CAD build for the part. Positions are in the model's coordinates, mm. A direction names the side the tool comes from. Round coordinates to 2 decimals unless told otherwise and drop trailing zeros. Loops run counter-clockwise (first coordinate to the right, second up) from the corner with the lowest first, then second, coordinate; pieces in that order, holes last.
```python
from build123d import *

# Parameters (mm, degrees)
BOSS_EXTRUDE1_DEPTH = 50
SKETCH2_W           = 3
SKETCH2_H           = 45
CUT_EXTRUDE1_DEPTH  = 50
SKETCH3_W           = 2
SKETCH3_H           = 45
CUT_EXTRUDE2_DEPTH  = 83.643814046
SKETCH4_W           = 3
SKETCH4_H           = 2
BOSS_EXTRUDE2_DEPTH = 39
SKETCH5_W           = 8
SKETCH5_H           = 2
BOSS_EXTRUDE3_DEPTH = 39
CUT_EXTRUDE3_REACH  = 83.222
SKETCH6_R           = 2.5


with BuildPart() as part:
    # Sketch1 → Boss-Extrude1 (new body)
    with BuildSketch(Plane.XY):
        Polygon((-8, 8), (53, 8), (53, -31), (-8, -31), (-8, -23.5), (-8, 0.5), align=None)
        Polygon((0, 0), (45, 0), (45, -23), (0, -23), (0, -15.5), (-3, -15.5), (-3, -7.5), (0, -7.5), align=None, mode=Mode.SUBTRACT)
    extrude(amount=BOSS_EXTRUDE1_DEPTH)

    # Sketch2 → Cut-Extrude1 (cut)
    with BuildSketch(Plane(origin=(0, 8, 0), x_dir=(1, 0, 0), z_dir=(0, 1, 0))):
        with Locations((-6.5, -24.5)):
            Rectangle(SKETCH2_W, SKETCH2_H)
        with Locations((51.5, -24.5)):
            Rectangle(SKETCH2_W, SKETCH2_H)
    extrude(amount=-CUT_EXTRUDE1_DEPTH, mode=Mode.SUBTRACT)

    # Sketch3 → Cut-Extrude2 (cut, through all)
    with BuildSketch(Plane(origin=(0, 8, 0), x_dir=(1, 0, 0), z_dir=(0, 1, 0))):
        with Locations((49, -24.5)):
            Rectangle(SKETCH3_W, SKETCH3_H)
    extrude(amount=-CUT_EXTRUDE2_DEPTH, mode=Mode.SUBTRACT)

    # Sketch4 → Boss-Extrude2 (add)
    with BuildSketch(Plane(origin=(0, 8, 0), x_dir=(1, 0, 0), z_dir=(0, 1, 0))):
        with Locations((54.5, -1)):
            Rectangle(SKETCH4_W, SKETCH4_H)
    extrude(amount=-BOSS_EXTRUDE2_DEPTH)

    # Sketch5 → Boss-Extrude3 (add)
    with BuildSketch(Plane(origin=(0, 8, 0), x_dir=(1, 0, 0), z_dir=(0, 1, 0))):
        with Locations((-9, -1)):
            Rectangle(SKETCH5_W, SKETCH5_H)
    extrude(amount=-BOSS_EXTRUDE3_DEPTH)

    # Sketch6 → Cut-Extrude3 (cut, up to next)
    with BuildSketch(Plane(origin=(0, 0, 0), x_dir=(-1, 0, 0), z_dir=(0, 0, -1)), mode=Mode.PRIVATE) as cut_extrude3_sk1:
        with Locations((-52, -1.5)):
            Circle(SKETCH6_R)
    cut_extrude3_tool1 = extrude(cut_extrude3_sk1.sketch, amount=-CUT_EXTRUDE3_REACH, mode=Mode.PRIVATE) & part.part
    # Sketch6 → Cut-Extrude3 (cut, up to next)
    with BuildSketch(Plane(origin=(0, 0, 0), x_dir=(-1, 0, 0), z_dir=(0, 0, -1)), mode=Mode.PRIVATE) as cut_extrude3_sk2:
        with Locations((-52, -21.5)):
            Circle(SKETCH6_R)
    cut_extrude3_tool2 = extrude(cut_extrude3_sk2.sketch, amount=-CUT_EXTRUDE3_REACH, mode=Mode.PRIVATE) & part.part
    # Sketch6 → Cut-Extrude3 (cut, up to next)
    with BuildSketch(Plane(origin=(0, 0, 0), x_dir=(-1, 0, 0), z_dir=(0, 0, -1)), mode=Mode.PRIVATE) as cut_extrude3_sk3:
        with Locations((9, -21.5)):
            Circle(SKETCH6_R)
    cut_extrude3_tool3 = extrude(cut_extrude3_sk3.sketch, amount=-CUT_EXTRUDE3_REACH, mode=Mode.PRIVATE) & part.part
    # Sketch6 → Cut-Extrude3 (cut, up to next)
    with BuildSketch(Plane(origin=(0, 0, 0), x_dir=(-1, 0, 0), z_dir=(0, 0, -1)), mode=Mode.PRIVATE) as cut_extrude3_sk4:
        with Locations((9, -1.5)):
            Circle(SKETCH6_R)
    cut_extrude3_tool4 = extrude(cut_extrude3_sk4.sketch, amount=-CUT_EXTRUDE3_REACH, mode=Mode.PRIVATE) & part.part
    add(cut_extrude3_tool1.solids().sort_by_distance((52, -1.5, 0))[0], mode=Mode.SUBTRACT)
    add(cut_extrude3_tool2.solids().sort_by_distance((52, -21.5, 0))[0], mode=Mode.SUBTRACT)
    add(cut_extrude3_tool3.solids().sort_by_distance((-9, -21.5, 0))[0], mode=Mode.SUBTRACT)
    add(cut_extrude3_tool4.solids().sort_by_distance((-9, -1.5, 0))[0], mode=Mode.SUBTRACT)


solid = part.part
```
Item 1: Cut at B-B, the plane x = -9. Give the cut face in (y, z).
Answers follow:
outline: (-31, 0) - (-24, 0) - (-24, 2) - (-31, 2) - close; (-19, 0) - (-4, 0) - (-4, 2) - (-19, 2) - close; (1, 0) - (8, 0) - (8, 2) - (1, 2) - close
Item 2: Two-plate mould, pull along X, no slides. Class faces 1 (the flat face through (-7, -11, 47)), 2 (the cylindrical face through (49.69, -2.46, 0.99)), 3 (the flat face through (48, -11, 25)): released by +X, released by -X, zero draft, split by the parting line, or undercut.
Answers follow:
face 1: zero draft
face 2: undercut
face 3: released by +X
Item 3: Cut at D-D, the plane y = -1.5. Give the cut face in (x, z).
Answers follow:
outline: (-13, 0) - (-11.5, 0) - (-11.5, 2) - (-13, 2) - close; (-8, 47) - (-5, 47) - (-5, 2) - (-6.5, 2) - (-6.5, 0) - (0, 0) - (0, 50) - (-8, 50) - close; (45, 0) - (49.5, 0) - (49.5, 2) - (48, 2) - (48, 47) - (53, 47) - (53, 50) - (45, 50) - close; (54.5, 0) - (56, 0) - (56, 2) - (54.5, 2) - close
Item 4: Cut at A-A, the plane y = -14. Give the cut face in (x, z), plus the area to 3 significant figures.
Answers follow:
outline: (-13, 0) - (-3, 0) - (-3, 50) - (-8, 50) - (-8, 47) - (-5, 47) - (-5, 2) - (-13, 2) - close; (45, 0) - (56, 0) - (56, 2) - (48, 2) - (48, 47) - (53, 47) - (53, 50) - (45, 50) - close
area: 306 mm2
Item 5: 3-axis set-ups, long thin cutter, end or side, ignore diameter. For faces 4 (the flat face through (52, -11, 2)), 5 (the flat face through (-5, -11, 25)), 6 (the flat face through (53, -11, 48)), 7 (the flat face through (0, -19, 25)), 8 (the flat face through (-8, -11, 48)): which of +Z, -Z, +X, -X, +Y, -Y reach the whole face in a straight line?
Answers follow:
face 4: +X, +Y, -Y
face 5: -X, +Y, -Y
face 6: +Z, +X, +Y, -Y
face 7: +Z, -Z
face 8: +Z, -X, +Y, -Y
Item 6: Probe line 1 (Y direction, x = -9, z = 0.4); line 2 (Y direction, x = 37, z = 26); line 3 (X direction, y = -19, z = 23). List the from-to ranges inside material, lowest first.
Answers follow:
line 1: y = -31 to -24, -19 to -4, 1 to 8
line 2: y = -31 to -23, 0 to 8
line 3: x = -5 to 0, 45 to 48
Item 7: Cut at C-C, the plane x = 52. Give the cut face in (y, z), plus the area to 3 significant figures.
Answers follow:
outline: (-31, 0) - (-24, 0) - (-24, 2) - (-31, 2) - close; (-31, 47) - (8, 47) - (8, 50) - (-31, 50) - close; (-19, 0) - (-4, 0) - (-4, 2) - (-19, 2) - close; (1, 0) - (8, 0) - (8, 2) - (1, 2) - close
area: 175 mm2
Item 8: Flat gauge pins, fed straight in: P1, Ø6.5, axis at x = -9, y = -18.5, coming from the +Z side; P2, Ø19.5, axis at y = -12.5, z = 13.5, coming from the +X side; P3, Ø3, axis at y = -26.5, z = 15.5, coming from the -X side; P4, Ø3.5, axis at y = -12, z = 48.5, coming from the -X side. Where does each tip first touch, or does it go through?
Answers follow:
P1: stops at z = 50
P2: stops at x = 48
P3: stops at x = -5
P4: stops at x = -8
